Input: part model. Units: mm. Frame: model coordinates. Face numbers are marked on the shaded views. Give positions to 0.01 mm unless a question says otherwise; leave off trailing zeros. Loops run counter-clockwise (first coordinate to the right, second up) from the corner with the lowest first, then second, coordinate; pieces in that order, holes last. Notation, with made-up numbers: (59.5, 71.25) - (63.5, 71.25) arc R24 cw to (63.5, 88.25) - close; hole circle Ø2 at (56.5, -0.5). An arc over 180 degrees is marked (long way). Answer as a JSON object with one key per item and string values.
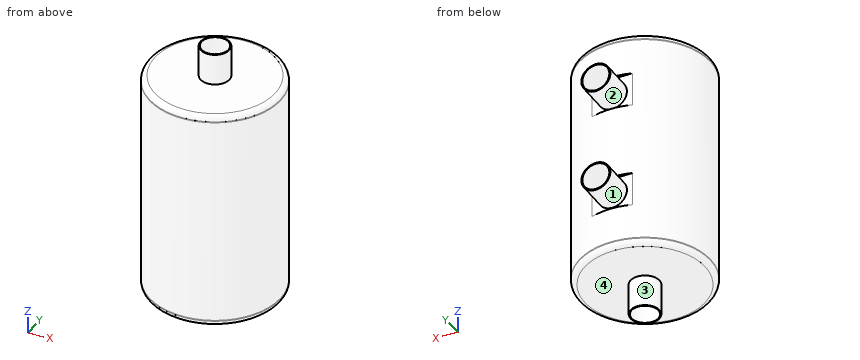
from build123d import *

# Parameters (mm, degrees)
SKETCH2_R               = 31
SKETCH2_R_2             = 28
BOSS_EXTRUDE1_DEPTH     = 100
SKETCH3_R               = 31
BOSS_EXTRUDE2_DEPTH     = 3
SKETCH4_R               = 31
BOSS_EXTRUDE3_DEPTH     = 3
SKETCH5_W               = 16
SKETCH5_H               = 1.5
CUT_EXTRUDE1_DEPTH      = 32
CUT_EXTRUDE1_DEPTH_BACK = 32
SKETCH6_R               = 6.85
SKETCH6_R_2             = 6.35
BOSS_EXTRUDE4_DEPTH     = 15
SKETCH6_2_R             = 6.35
CUT_EXTRUDE2_DEPTH      = 15
SKETCH7_R               = 6.85
SKETCH7_R_2             = 6.35
BOSS_EXTRUDE5_DEPTH     = 15
SKETCH7_2_R             = 6.35
CUT_EXTRUDE3_DEPTH      = 15
FILLET1_R               = 2.5


with BuildPart() as part:
    # Sketch2 → Boss-Extrude1 (new body)
    with BuildSketch(Plane.XY):
        Circle(SKETCH2_R)
        Circle(SKETCH2_R_2, mode=Mode.SUBTRACT)
    extrude(amount=-BOSS_EXTRUDE1_DEPTH)

    # Sketch3 → Boss-Extrude2 (add)
    with BuildSketch(Plane.XY):
        Circle(SKETCH3_R)
    extrude(amount=BOSS_EXTRUDE2_DEPTH)

    # Sketch4 → Boss-Extrude3 (add)
    with BuildSketch(Plane(origin=(0, 0, -100), x_dir=(-1, 0, 0), z_dir=(0, 0, -1))):
        Circle(SKETCH4_R)
    extrude(amount=BOSS_EXTRUDE3_DEPTH)

    # Sketch5 → Cut-Extrude1 (cut, two sides)
    with BuildSketch(Plane(origin=(0, 0, 0), x_dir=(0, 0, -1), z_dir=(1, 0, 0))) as cut_extrude1_sk:
        with Locations((75.269911272, 30.25)):
            Rectangle(SKETCH5_W, SKETCH5_H)
        with Locations((24.730088728, 30.25)):
            Rectangle(SKETCH5_W, SKETCH5_H)
    extrude(amount=CUT_EXTRUDE1_DEPTH, mode=Mode.SUBTRACT)
    extrude(cut_extrude1_sk.sketch, amount=-CUT_EXTRUDE1_DEPTH_BACK, mode=Mode.SUBTRACT)

    # Sketch6 → Boss-Extrude4 (add)
    with BuildSketch(Plane(origin=(0, 29.5, 0), x_dir=(1, 0, 0), z_dir=(0, 1, 0))):
        with Locations((0, 25)):
            Circle(SKETCH6_R)
        with Locations((0, 25)):
            Circle(SKETCH6_R_2, mode=Mode.SUBTRACT)
        with Locations((0, 75)):
            Circle(SKETCH6_R)
        with Locations((0, 75)):
            Circle(SKETCH6_R_2, mode=Mode.SUBTRACT)
    extrude(amount=BOSS_EXTRUDE4_DEPTH)

    # Sketch6<2> → Cut-Extrude2 (cut)
    with BuildSketch(Plane(origin=(0, 29.5, 0), x_dir=(1, 0, 0), z_dir=(0, 1, 0))):
        with Locations((0, 25)):
            Circle(SKETCH6_2_R)
        with Locations((0, 75)):
            Circle(SKETCH6_2_R)
    extrude(amount=-CUT_EXTRUDE2_DEPTH, mode=Mode.SUBTRACT)

    # Sketch7 → Boss-Extrude5 (add)
    with BuildSketch(Plane.XY.offset(3)):
        Circle(SKETCH7_R)
        Circle(SKETCH7_R_2, mode=Mode.SUBTRACT)
    boss_extrude5 = extrude(amount=BOSS_EXTRUDE5_DEPTH)

    # Sketch7<2> → Cut-Extrude3 (cut)
    with BuildSketch(Plane.XY.offset(3)):
        Circle(SKETCH7_2_R)
    cut_extrude3 = extrude(amount=-CUT_EXTRUDE3_DEPTH, mode=Mode.SUBTRACT)

    # Mirror2: Boss-Extrude5, Cut-Extrude3 across plane
    add(boss_extrude5.mirror(Plane.XY.offset(-50)))
    add(cut_extrude3.mirror(Plane.XY.offset(-50)), mode=Mode.SUBTRACT)

    # Fillet1
    fillet1_edges = [part.edges().sort_by_distance(p)[0] for p in [
        (-31, 0, 3),
        (31, 0, -103),
    ]]
    fillet(fillet1_edges, radius=FILLET1_R)


solid = part.part
Item 1: Material intervals for line 1 (Z direction, x = 0, y = 41.5); line 2 (X direction, y = -1, z = -45.5); line 3 (Z direction, x = -15, y = -22.5), sorted ascending. Write a range as [from, to].
Geometry check:
{"line 1": "z = [-81.85, -81.35], [-68.65, -68.15], [-31.85, -31.35], [-18.65, -18.15]", "line 2": "x = [-30.98, -27.98], [27.98, 30.98]", "line 3": "z = [-103, -100], [0, 3]"}
Item 2: Cut plane D-D (z = -106.5). Return loops of the section in (x, y).
Geometry check:
{"outline": "circle Ø13.7 at (0, 0); hole circle Ø12.7 at (0, 0)"}
Item 3: Mould query, pull axis Z, two halves, no side actions, for the marked faces 1, 2, 3 and 4. Classes: released by +Z, released by -Z, zero draft, split by the parting line, or undercut.
Geometry check:
{"face 1": "undercut", "face 2": "undercut", "face 3": "zero draft", "face 4": "released by -Z"}
Item 4: Cut plane A-A (y = 0). Return loops of the section in (x, z).
Geometry check:
{"outline": "(-31, -100.5) arc R2.5 ccw to (-28.5, -103) - (-6.85, -103) - (-6.85, -118) - (-6.35, -118) - (-6.35, -100) - (-28, -100) - (-28, 0) - (-6.35, 0) - (-6.35, 18) - (-6.85, 18) - (-6.85, 3) - (-28.5, 3) arc R2.5 ccw to (-31, 0.5) - close; (6.35, -118) - (6.85, -118) - (6.85, -103) - (28.5, -103) arc R2.5 ccw to (31, -100.5) - (31, 0.5) arc R2.5 ccw to (28.5, 3) - (6.85, 3) - (6.85, 18) - (6.35, 18) - (6.35, 0) - (28, 0) - (28, -100) - (6.35, -100) - close"}
Item 5: Cut plane C-C (z = -25). Return loops of the section in (x, y).
Geometry check:
{"outline": "(-9.53, 29.5) arc R31 ccw (long way) to (9.53, 29.5) - (6.85, 29.5) - (6.85, 44.5) - (6.35, 44.5) - (6.35, 27.27) arc R28 cw (long way) to (-6.35, 27.27) - (-6.35, 44.5) - (-6.85, 44.5) - (-6.85, 29.5) - close"}
Item 6: Cut plane B-B (z = -3.5). Return loops of the section in (x, y).
Geometry check:
{"outline": "circle Ø62 at (0, 0); hole circle Ø56 at (0, 0)"}
Item 7: Contact query for flat-ended pins moving along their axis: P1, Ø4, axis at x = -20.5, y = -21, coming from the +Z side; P2, Ø2, axis at x = 14.5, z = -45, coming from the +Y side; P3, Ø6, axis at x = 13, z = -8.5, coming from the +Y side. Output: stop coordinate, or through.
Geometry check:
{"P1": "stops at z = 3", "P2": "stops at y = 27.91", "P3": "stops at y = 29.34"}
